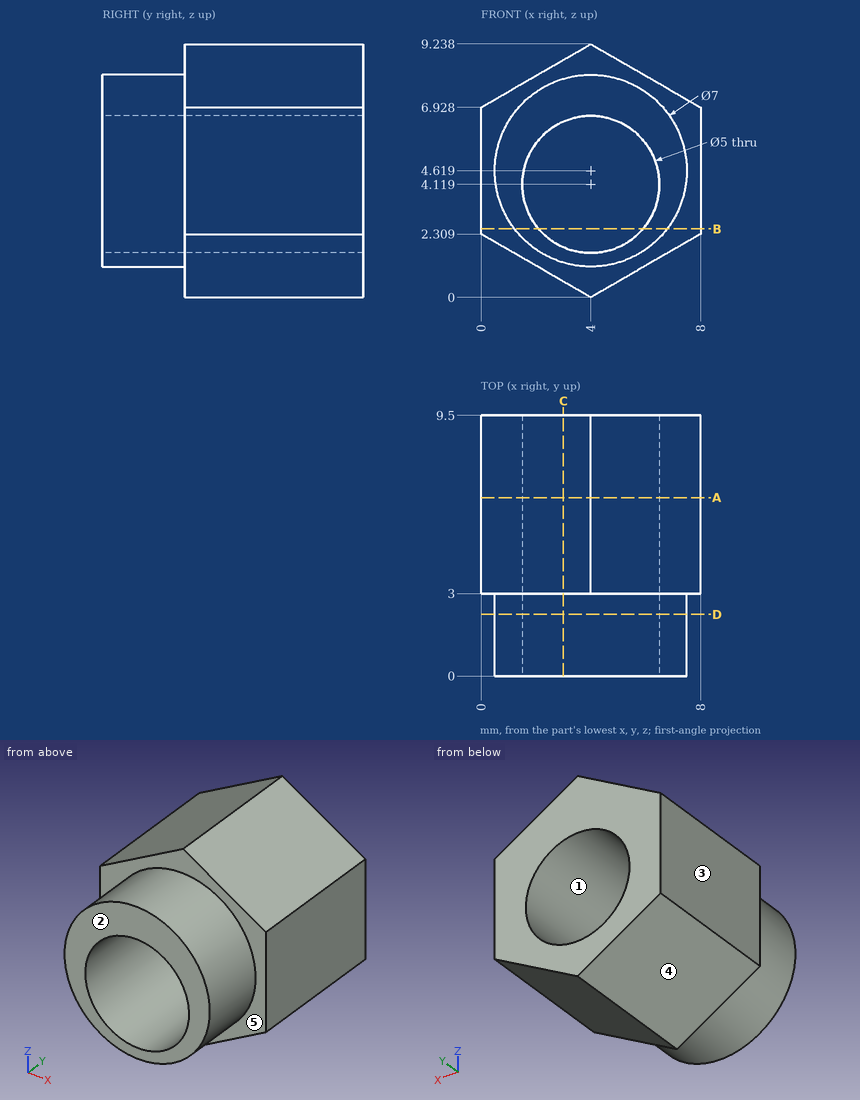
Part print with two shaded views. Sizes in mm from the minimum x, y, z corner. A direction names the side the tool comes from. Coordinates: 2 decimals unless noted, no trailing zeros. Order: outer loops, then holes, each group sorted by start corner. A loop starts at its lowest first (then second) coordinate and runs counter-clockwise, first axis right, second up. Notation, with made-up numbers: (56, 74) - (98, 74) arc R19 cw to (98, 105) - close; hole circle Ø1 at (52.5, 40). An arc over 180 degrees is marked (long way). Write item = value, one per line. Start each with the question number.
1) Saw through at A-A on y = 6.5. Write the cut outline in (x, z), then the cut area to 3 significant figures.
2) Flat gauge pins, fed straight in: pin 1 Ø2 at (x, y) = (6, 3) entering from +Z; pin 2 Ø2 at (x, z) = (4, 5.5) entering from +Y. Where does each tip first touch, or does it go through?
3) Saw through at B-B on z = 2.5. Write the cut outline in (x, y) (1 decimal).
4) Wall check: line 1 along X through (y, z) = (8.25, 4); line 2 along X through (y, z) = (3.75, 4.75); line 3 along Z through (x, y) = (5.5, 1) (1 decimal). Give the ranges that are in metal, low to high. Write a range as from..to.
5) 3-axis set-ups, long thin cutter, end or side, ignore diameter. For the marked faces 4 and 5: which of +Z, -Z, +X, -X, +Y, -Y reach the whole face in a straight line?
6) Saw through at C-C on x = 3. Write the cut outline in (y, z) (1 decimal).
7) Two-plate mould, pull along X, no slides. Class the marked faces 1, 2 and 3: pulls with the +X half, pulls with the -X half, needs draft (parallel to the pull), parting line crosses it, or undercut.
8) Saw through at D-D on y = 2.25. Write the cut outline in (x, z).
From the geometry:
q1.outline = (0, 2.31) - (4, 0) - (8, 2.31) - (8, 6.93) - (4, 9.24) - (0, 6.93) - close; hole circle Ø5 at (4, 4.12)
q1.area = 35.8 mm^2
q2.pin_1 = 8.66
q2.pin_2 = through
q3.outline = (0, 3) - (1.2, 3) - (1.2, 0) - (2.1, 0) - (2.1, 9.5) - (0, 9.5) - close; (5.9, 0) - (6.8, 0) - (6.8, 3) - (8, 3) - (8, 9.5) - (5.9, 9.5) - close
q4.line_1 = 0..1.5, 6.5..8
q4.line_2 = 0..1.58, 6.42..8
q4.line_3 = 1.5..2.1, 6.1..7.8
q5.face_4 = -Z, -X, +Y, -Y
q5.face_5 = -Y
q6.outline = (0, 1.3) - (3, 1.3) - (3, 0.6) - (9.5, 0.6) - (9.5, 1.8) - (0, 1.8) - close; (0, 6.4) - (9.5, 6.4) - (9.5, 8.7) - (3, 8.7) - (3, 8) - (0, 8) - close
q7.face_1 = undercut
q7.face_2 = needs draft
q7.face_3 = pulls with the -X half
q8.outline = circle Ø7 at (4, 4.62); hole circle Ø5 at (4, 4.12)
